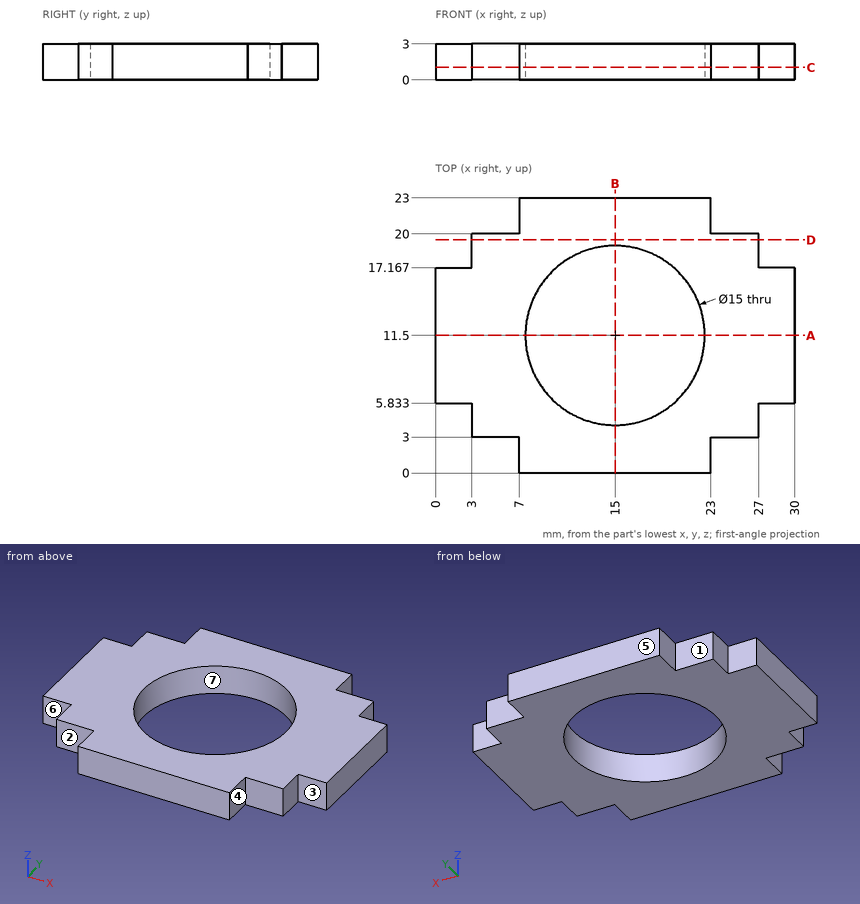
Can you work these out from the drawing? Everything is in mm from the part's minimum corner. A direction names the side the tool comes from. Give positions to 0.01 mm unless a question says otherwise; leave off trailing zeros. Loops run counter-clockwise (first coordinate to the right, second up) from the corner with the lowest first, then second, coordinate; pieces in that order, holes last. Notation, with made-up numbers: (30, 88) -> (46, 88) arc R25 cw to (46, 109) -> close; hole circle Ø9 at (-10.75, 20.5). An arc over 180 degrees is marked (long way). Put each result on its own line as item: value.
(1) Imagine slicing it at A-A on y = 11.5. Write out the boundary of the cut face in (x, z), plus the area to 3 significant figures.
Computed:
outline: (0, 0) -> (7.5, 0) -> (7.5, 3) -> (0, 3) -> close; (22.5, 0) -> (30, 0) -> (30, 3) -> (22.5, 3) -> close
area: 45.0 mm^2
(2) I'm going to push flat-ended pins straight in: pin 1 Ø0.9 at (x, z) = (1, 1.5) entering from +Y; pin 2 Ø1.5 at (x, z) = (24.5, 1) entering from -Y; pin 3 Ø1.5 at (x, z) = (29, 1.5) entering from -Y; pin 4 Ø12 at (x, y) = (21, 13.5) entering from -Z. Where does each tip first touch, or does it pass through?
Computed:
pin 1: y = 17.17
pin 2: y = 3
pin 3: y = 5.83
pin 4: z = 0
(3) Imagine slicing it at C-C on z = 1.05. Write out the boundary of the cut face in (x, y).
Computed:
outline: (0, 5.83) -> (3, 5.83) -> (3, 3) -> (7, 3) -> (7, 0) -> (23, 0) -> (23, 3) -> (27, 3) -> (27, 5.83) -> (30, 5.83) -> (30, 17.17) -> (27, 17.17) -> (27, 20) -> (23, 20) -> (23, 23) -> (7, 23) -> (7, 20) -> (3, 20) -> (3, 17.17) -> (0, 17.17) -> close; hole circle Ø15 at (15, 11.5)
(4) Thinking about a two-plate mould opening in Y: for the marked faces 4, 5, 6 and 7, which applies, pulls with the +Y half, pulls with the -Y half, needs draft (parallel to the pull), parting line crosses it, or undercut?
Computed:
face 4: needs draft
face 5: pulls with the +Y half
face 6: pulls with the -Y half
face 7: undercut
(5) Imagine slicing it at D-D on y = 19.5. Write out the boundary of the cut face in (x, z).
Computed:
outline: (3, 0) -> (27, 0) -> (27, 3) -> (3, 3) -> close
(6) Please list where these lines run through material, in increasing order: probe 1 along Y at (x, z) = (15, 0.75); probe 2 along X at (y, z) = (20.25, 1.55); probe 3 along Y at (x, z) = (25.5, 2.85). Write a range as [from, to].
Computed:
probe 1: [0, 4], [19, 23]
probe 2: [7, 23]
probe 3: [3, 20]
(7) For the marked faces 1, 2 and 3, which set-ups out of +Z, -Z, +X, -X, +Y, -Y let a thin tool reach every point of the face, with its end or its side?
Computed:
face 1: +Z, -Z, -X, +Y
face 2: +Z, -Z, -X, -Y
face 3: +Z, -Z, +X, -Y
(8) Imagine slicing it at B-B on x = 15. Write out the boundary of the cut face in (y, z).
Computed:
outline: (0, 0) -> (4, 0) -> (4, 3) -> (0, 3) -> close; (19, 0) -> (23, 0) -> (23, 3) -> (19, 3) -> close
